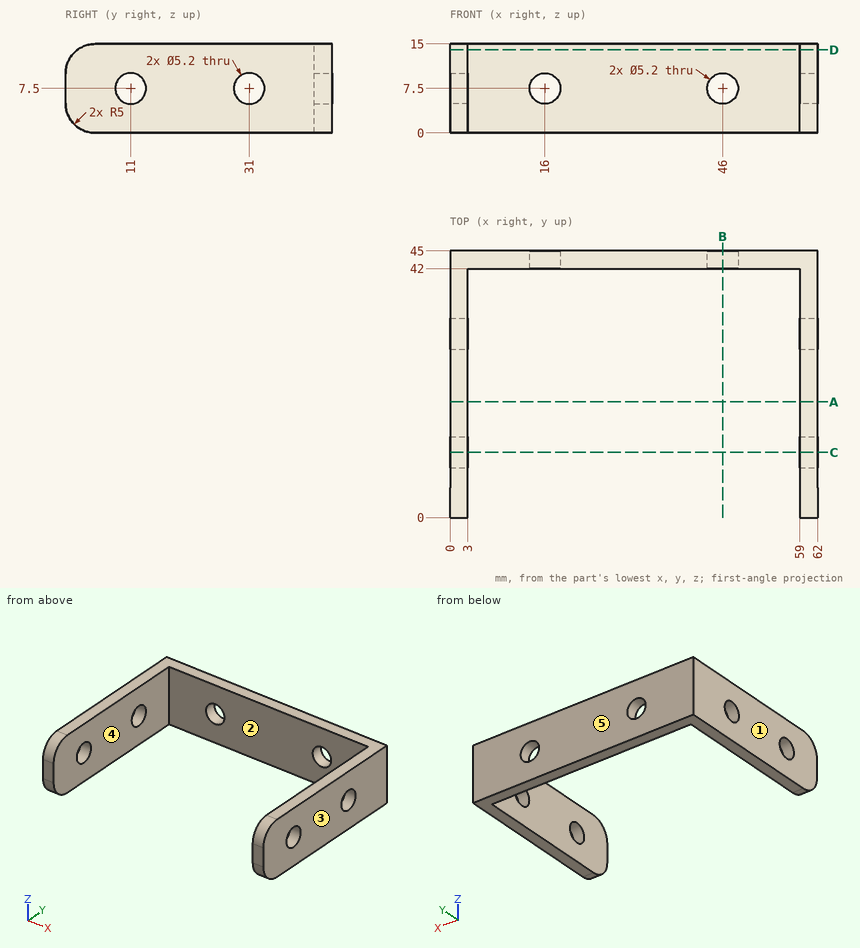
The drawing under review shows one solid part. Ordinate dimensions are in mm from its lowest x, y, z. A direction names the side the tool comes from. Coordinates: 2 decimals unless noted, no trailing zeros. Write each loop counter-clockwise with the first axis right and the second up, starting at its lowest first coordinate (ties: lowest second). Pieces come first, ordered by that corner, then holes. Notation, with made-up numbers: M -23,74.25 L 18,74.25 A12 cw 18,93.25 Z; hole C 57,69 d2. An arc over 180 degrees is marked long. Put each result on its own line as item: value.
1) Draft analysis for pull direction X (two halves, no side actions). For the marked faces 1, 2 and 3, state which applies: released by +X, released by -X, zero draft, split by the parting line, or undercut.
Computed:
face 1: released by -X
face 2: undercut
face 3: released by +X
2) Add section B-B on x = 46. Give the boundary of the cut face in (y, z), then the cut area to 3 significant figures.
Computed:
outline: M 42,0 L 45,0 L 45,4.9 L 42,4.9 Z; M 42,10.1 L 45,10.1 L 45,15 L 42,15 Z
area: 29.4 mm2
3) Wall thickness on probe 1 along Y at (x, z) = (60.2, 7.5); probe 2 along X at (y, z) = (24.5, 9.5); probe 3 along Z at (x, y) = (16, 42.9): over which ranges is each line inside the solid? List them lowest first. Write a range as [from, to].
Computed:
probe 1: y = [0, 8.4], [13.6, 28.4], [33.6, 45]
probe 2: x = [0, 3], [59, 62]
probe 3: z = [0, 4.9], [10.1, 15]
4) Clearance check with flat-ended pins moving along their axes: pin 1 Ø3 at (x, z) = (16, 11) entering from -Y; pin 2 Ø4.5 at (x, z) = (46, 7.5) entering from -Y. State where each tip first meets the part, or that it passes through.
Computed:
pin 1: stops at y = 42
pin 2: passes through
5) Add section D-D on z = 14. Give the boundary of the cut face in (x, y), then the cut area to 3 significant figures.
Computed:
outline: M 0,2 L 3,2 L 3,42 L 59,42 L 59,2 L 62,2 L 62,45 L 0,45 Z
area: 426 mm2
6) For the marked faces 4 and 5, list the 3-axis set-ups (+Z, -Z, +X, -X, +Y, -Y) from which the entire face can be reached by the end or side of a thin tool; tool diameter is ignored.
Computed:
face 4: +Z, -Z, -Y
face 5: +Z, -Z, +X, -X, +Y
7) Add section C-C on y = 11. Give the boundary of the cut face in (x, z), then the cut area to 3 significant figures.
Computed:
outline: M 0,0 L 3,0 L 3,4.9 L 0,4.9 Z; M 0,10.1 L 3,10.1 L 3,15 L 0,15 Z; M 59,0 L 62,0 L 62,4.9 L 59,4.9 Z; M 59,10.1 L 62,10.1 L 62,15 L 59,15 Z
area: 58.8 mm2
8) Add section A-A on y = 19.5. Give the boundary of the cut face in (x, z), then the cut area to 3 significant figures.
Computed:
outline: M 0,0 L 3,0 L 3,15 L 0,15 Z; M 59,0 L 62,0 L 62,15 L 59,15 Z
area: 90.0 mm2
